from build123d import *

# Parameters (mm, degrees)
F0_R     = 1.7526
F1_DEPTH = 5.842


with BuildPart() as f1:
    # F0 (on Front) → F1 (new body)
    with BuildSketch(Plane.XZ):
        with BuildLine():
            ThreePointArc((25.4, 0), (0, 25.4), (-25.4, 0))
            Line((-25.4, 0), (-25.4, -35.56))
            Line((-25.4, -35.56), (-16.2526, -35.56))
            Line((-16.2526, -35.56), (-16.2526, -32.385))
            Line((-16.2526, -32.385), (-18.46875, -32.385))
            Line((-18.46875, -32.385), (-18.46875, -29.606875))
            Line((-18.46875, -29.606875), (-16.2526, -29.606875))
            Line((-16.2526, -29.606875), (-16.2526, -28.019375))
            Line((-16.2526, -28.019375), (-12.7474, -28.019375))
            Line((-12.7474, -28.019375), (-12.7474, -29.606875))
            Line((-12.7474, -29.606875), (-10.53125, -29.606875))
            Line((-10.53125, -29.606875), (-10.53125, -32.385))
            Line((-10.53125, -32.385), (-12.7474, -32.385))
            Line((-12.7474, -32.385), (-12.7474, -35.56))
            Line((-12.7474, -35.56), (-6.35, -35.56))
            Line((-6.35, -35.56), (-6.35, -41.402))
            Line((-6.35, -41.402), (6.35, -41.402))
            Line((6.35, -41.402), (6.35, -35.56))
            Line((6.35, -35.56), (12.7474, -35.56))
            Line((12.7474, -35.56), (12.7474, -32.385))
            Line((12.7474, -32.385), (10.53125, -32.385))
            Line((10.53125, -32.385), (10.53125, -29.606875))
            Line((10.53125, -29.606875), (12.7474, -29.606875))
            Line((12.7474, -29.606875), (12.7474, -28.019375))
            Line((12.7474, -28.019375), (16.2526, -28.019375))
            Line((16.2526, -28.019375), (16.2526, -29.606875))
            Line((16.2526, -29.606875), (18.46875, -29.606875))
            Line((18.46875, -29.606875), (18.46875, -32.385))
            Line((18.46875, -32.385), (16.2526, -32.385))
            Line((16.2526, -32.385), (16.2526, -35.56))
            Line((16.2526, -35.56), (25.4, -35.56))
            Line((25.4, -35.56), (25.4, 0))
        make_face()
        with Locations((0, -9)):
            Circle(F0_R, mode=Mode.SUBTRACT)
        with Locations((-9, 0)):
            Circle(F0_R, mode=Mode.SUBTRACT)
        with Locations((0, 9)):
            Circle(F0_R, mode=Mode.SUBTRACT)
        with Locations((9, 0)):
            Circle(F0_R, mode=Mode.SUBTRACT)
    extrude(amount=F1_DEPTH)


solid = f1.part
The model under review builds one solid part; all positions refer to its coordinate system, in mm. A direction names the side the tool comes from. Give positions to 0.01 mm unless a question says otherwise; leave off trailing zeros. Loops run counter-clockwise (first coordinate to the right, second up) from the corner with the lowest first, then second, coordinate; pieces in that order, holes last. Notation, with made-up numbers: (66.25, 26.5) -> (70.25, 26.5) arc R30 cw to (70.25, 50.5) -> close; hole circle Ø6 at (32, 50.5). An arc over 180 degrees is marked (long way). Put each result on its own line as item: value. Start each with the question number.
1. Mouldability with a two-part tool opening along Z and no side actions: class faces 1 (the face through (-6.35, -3, -38)), 2 (the face through (-10, -3, -35.56)), 3 (the face through (-17, -3, -32.385)) as released by +Z, released by -Z, zero draft, split by the parting line, or undercut.
2. We need section A-A on x = 0. State the section outline as (y, z) points, then the cut area to 3 significant figures.
3. We need section B-B on z = -9. State the section outline as (x, y) points, then the cut area to 3 significant figures.
4. We need section D-D on x = 9. State the section outline as (y, z) points.
5. Wall thickness on probe 1 along Z at (x, y) = (0, -2.6); probe 2 along Z at (x, y) = (1.5, -2); probe 3 along Z at (x, y) = (8.5, -5): over which ranges is each line inside the solid? List them lowest first.
6. Clearance check with flat-ended pins moving along their axes: P1, Ø5.5, axis at x = 9, z = 0, coming from the -Y side; P2, Ø2.5, axis at x = -17, y = -1.5, coming from the -Z side; P3, Ø1.5, axis at x = 14, z = -34, coming from the +Y side. State where each tip first meets the part, or that it passes through.
7. We need section C-C on y = -2.4. State how many separate pieces and enclosed holes the cut face has, then the cut area to 3 significant figures.
8. For faces 4 (the face through (-21, -3, -35.56)), 5 (the face through (-12.747, -3, -34)), 6 (the face through (5, 0, -8)), 7 (the face through (12, -3, -29.607)), 8 (the face through (21, -3, -35.56)), list the 3-axis set-ups (+Z, -Z, +X, -X, +Y, -Y) from which the entire face can be reached by the end or side of a thin tool; tool diameter is ignored.
Determined:
1. face 1: zero draft
1. face 2: released by -Z
1. face 3: undercut
2. outline: (-5.84, -41.4) -> (0, -41.4) -> (0, -10.75) -> (-5.84, -10.75) -> close; (-5.84, -7.25) -> (0, -7.25) -> (0, 7.25) -> (-5.84, 7.25) -> close; (-5.84, 10.75) -> (0, 10.75) -> (0, 25.4) -> (-5.84, 25.4) -> close
2. area: 349 mm^2
3. outline: (-25.4, -5.84) -> (-1.75, -5.84) -> (-1.75, 0) -> (-25.4, 0) -> close; (1.75, -5.84) -> (25.4, -5.84) -> (25.4, 0) -> (1.75, 0) -> close
3. area: 276 mm^2
4. outline: (-5.84, -35.56) -> (0, -35.56) -> (0, -1.75) -> (-5.84, -1.75) -> close; (-5.84, 1.75) -> (0, 1.75) -> (0, 23.75) -> (-5.84, 23.75) -> close
5. probe 1: -41.4 to -10.75, -7.25 to 7.25, 10.75 to 25.4
5. probe 2: -41.4 to -9.91, -8.09 to 8.09, 9.91 to 25.36
5. probe 3: -35.56 to -1.68, 1.68 to 23.94
6. P1: y = -5.84
6. P2: z = -35.56
6. P3: through
7. separate pieces: 1
7. enclosed holes: 4
7. area: 2,780 mm^2
8. face 4: -Z, -X, +Y, -Y
8. face 5: -Z, +Y, -Y
8. face 6: +Z, -Z, +X, -X, +Y
8. face 7: +Y, -Y
8. face 8: -Z, +X, +Y, -Y
